Autodesk Inventor part; units mm, degrees
ref_plane "YZ Plane" through (0, 0, 0) normal (1, 0, 0) x (0, 1, 0)
ref_plane "XZ Plane" through (0, 0, 0) normal (0, 1, 0) x (-1, 0, 0)
ref_plane "XY Plane" through (0, 0, 0) normal (0, 0, 1) x (1, 0, 0)
sketch "Sketch1" plane through (0, 0, 0) normal (0, 0, 1) x (1, 0, 0)
  circle A0 centre (0, 0) radius 25.4
  circle A1 centre (0, 0) radius 31.75
  dimension "d1" = 50.8
  dimension "d2" = 6.35
extrude "Ring" add sketch "Sketch1" against normal blind 19.05
extrude "Back" add sketch "Sketch1" along normal blind 6.35 contours A0 | A1
sketch "Sketch2" plane through (0, 0, 6.35) normal (0, 0, 1) x (1, 0, 0)
  circle A0 centre (0, 0) radius 3.175
  circle A1 centre (-12.7, 0) radius 3.175
  circle A2 centre (12.7, 0) radius 3.175
  line L0 (-12.7, 0) -> (12.7, 0) construction
  dimension "d7" = 6.35
  dimension "d8" = 12.7
  dimension "d11" = 12.7
extrude "Holes" cut sketch "Sketch2" against normal through all
fillet "Fillets" radius 3.175 3 edges at (-31.75, 0, 6.35) (-31.75, 0, -19.05) (-25.4, 0, -19.05)
properties part number "friction-fit"
Here's how the part is built. I have some questions about the finished solid (model axes, mm). A direction names the side the tool comes from. Round coordinates to 2 decimals unless told otherwise and drop trailing zeros. Order: outer loops, then holes, each group sorted by start corner. A loop starts at its lowest first (then second) coordinate and runs counter-clockwise, first axis right, second up. Notation, with made-up numbers: (-14.5, -28) -> (-10.5, -28) arc R19 ccw to (-10.5, -13) -> close; hole circle Ø1 at (19.5, 17.25). An arc over 180 degrees is marked (long way). Use CSV: the item, a comma, the result in double quotes.
1. I'm going to push flat-ended pins straight in: P1, Ø5, axis at y = 11, z = -7.5, coming from the -X side; P2, Ø8.5, axis at x = -12.7, y = 0, coming from the -Z side; P3, Ø1, axis at x = -16.5, z = -15, coming from the -Y side. Where does each tip first touch, or does it pass through?
Recorded:
P1,"stops at x = -30.59"
P2,"stops at z = 0"
P3,"stops at y = -27.42"
2. I want a section at C-C on z = -13. List the corners of the cut face in (x, y) for me.
Recorded:
outline,"circle Ø63.5 at (0, 0); hole circle Ø50.8 at (0, 0)"
3. Which directions (+Z, -Z, +X, -X, +Y, -Y) give clear straight access to the entire face, cutting with the end or side of a thin tool? Please do faces 4 (the face through (5, 0, 0)), 5 (the face through (9.53, 0.14, 3.22)).
Recorded:
face 4,"-Z"
face 5,"+Z, -Z"
4. I want a section at B-B on y = 0. Give the number of separate pieces and of enclosed holes in the cut face, and give its area (3 significant figures).
Recorded:
separate pieces,"4"
enclosed holes,"0"
area,"511 mm2"
5. I need wall thicknesses on line 1 along Z through (x, y) = (-21, 1); line 2 along Y through (x, z) = (0, 3) (3 decimals); line 3 along X through (y, z) = (13, -8.75). Which ranges of each line are inside material? Lowest first, please.
Recorded:
line 1,"z = 0 to 6.35"
line 2,"y = -31.75 to -3.175, 3.175 to 31.75"
line 3,"x = -28.97 to -21.82, 21.82 to 28.97"
6. Thinking about a two-plate mould opening in X: for faces 1 (the face through (0, -6, 6.35)), 2 (the face through (-5.506, -24.796, -7.826)), 3 (the face through (-6.883, -30.995, -6.217)), which applies, pulls with the +X half, pulls with the -X half, needs draft (parallel to the pull), parting line crosses it, or undercut?
Recorded:
face 1,"needs draft"
face 2,"undercut"
face 3,"parting line crosses it"
